from build123d import *

# Parameters (mm, degrees)
CYLINDER1785_R     = 5
CYLINDER1785_DEPTH = 3
CYLINDER1786_R     = 2.5
CYLINDER1786_DEPTH = 20
CYLINDER1781_R     = 1.5
CYLINDER1781_DEPTH = 20
CYLINDER1783_R     = 1.5
CYLINDER1783_DEPTH = 20
CYLINDER1784_R     = 1.5
CYLINDER1784_DEPTH = 20
CYLINDER1782_R     = 1.5
CYLINDER1782_DEPTH = 20
BOX744_W           = 6
BOX744_H           = 6
BOX744_DEPTH       = 2
BOX746_W           = 6
BOX746_H           = 6
BOX746_DEPTH       = 2
BOX745_W           = 6
BOX745_H           = 6
BOX745_DEPTH       = 2
BOX742_W           = 6
BOX742_H           = 6
BOX742_DEPTH       = 2
BOX743_W           = 20
BOX743_H           = 80
BOX743_DEPTH       = 20
BOX747_W           = 38
BOX747_H           = 32
BOX747_DEPTH       = 26
CHAMFER060_SIZE    = 2


with BuildPart() as obj1:
    # Cylinder1785 → Cylinder1785 (new body)
    with BuildSketch(Plane(origin=(-112, 16, 66), x_dir=(0, 0, -1), z_dir=(1, 0, 0))):
        Circle(CYLINDER1785_R)
    extrude(amount=CYLINDER1785_DEPTH)


with BuildPart() as obj2:
    # Cylinder1786 → Cylinder1786 (new body)
    with BuildSketch(Plane(origin=(-117, 16, 66), x_dir=(0, 0, -1), z_dir=(1, 0, 0))):
        Circle(CYLINDER1786_R)
    extrude(amount=CYLINDER1786_DEPTH)


with BuildPart() as obj3:
    # Cylinder1781 → Cylinder1781 (new body)
    with BuildSketch(Plane(origin=(-83, 25, 54), x_dir=(1, 0, 0), z_dir=(0, 0, 1))):
        Circle(CYLINDER1781_R)
    extrude(amount=CYLINDER1781_DEPTH)


with BuildPart() as obj4:
    # Cylinder1783 → Cylinder1783 (new body)
    with BuildSketch(Plane(origin=(-109, 7, 54), x_dir=(1, 0, 0), z_dir=(0, 0, 1))):
        Circle(CYLINDER1783_R)
    extrude(amount=CYLINDER1783_DEPTH)


with BuildPart() as obj5:
    # Cylinder1784 → Cylinder1784 (new body)
    with BuildSketch(Plane(origin=(-109, 25, 54), x_dir=(1, 0, 0), z_dir=(0, 0, 1))):
        Circle(CYLINDER1784_R)
    extrude(amount=CYLINDER1784_DEPTH)


with BuildPart() as compound913:
    # Cylinder1782 → Cylinder1782 (new body)
    with BuildSketch(Plane(origin=(-83, 7, 54), x_dir=(1, 0, 0), z_dir=(0, 0, 1))):
        Circle(CYLINDER1782_R)
    extrude(amount=CYLINDER1782_DEPTH)

    # Compound913: union obj3, obj4, obj5
    add(obj3.part)
    add(obj4.part)
    add(obj5.part)


with BuildPart() as krychle744:
    # Box744 → Box744 (new body)
    with BuildSketch(Plane(origin=(-112, 22, 60), x_dir=(1, 0, 0), z_dir=(0, 0, 1))):
        with Locations((3, 3)):
            Rectangle(BOX744_W, BOX744_H)
    extrude(amount=BOX744_DEPTH)


with BuildPart() as krychle746:
    # Box746 → Box746 (new body)
    with BuildSketch(Plane(origin=(-86, 4, 60), x_dir=(1, 0, 0), z_dir=(0, 0, 1))):
        with Locations((3, 3)):
            Rectangle(BOX746_W, BOX746_H)
    extrude(amount=BOX746_DEPTH)


with BuildPart() as krychle745:
    # Box745 → Box745 (new body)
    with BuildSketch(Plane(origin=(-86, 22, 60), x_dir=(1, 0, 0), z_dir=(0, 0, 1))):
        with Locations((3, 3)):
            Rectangle(BOX745_W, BOX745_H)
    extrude(amount=BOX745_DEPTH)


with BuildPart() as compound912:
    # Box742 → Box742 (new body)
    with BuildSketch(Plane(origin=(-112, 4, 60), x_dir=(1, 0, 0), z_dir=(0, 0, 1))):
        with Locations((3, 3)):
            Rectangle(BOX742_W, BOX742_H)
    extrude(amount=BOX742_DEPTH)

    # Compound912: union Krychle744, Krychle746, Krychle745
    add(krychle744.part)
    add(krychle746.part)
    add(krychle745.part)


with BuildPart() as krychle743:
    # Box743 → Box743 (new body)
    with BuildSketch(Plane(origin=(-106, 4, 56), x_dir=(1, 0, 0), z_dir=(0, 0, 1))):
        with Locations((10, 40)):
            Rectangle(BOX743_W, BOX743_H)
    extrude(amount=BOX743_DEPTH)


with BuildPart() as chamfer060:
    # Box747 → Box747 (new body)
    with BuildSketch(Plane(origin=(-112, 0, 56), x_dir=(1, 0, 0), z_dir=(0, 0, 1))):
        with Locations((19, 16)):
            Rectangle(BOX747_W, BOX747_H)
    extrude(amount=BOX747_DEPTH)

    # Cut546: cut Krychle743
    add(krychle743.part, mode=Mode.SUBTRACT)

    # Cut547: cut Compound912
    add(compound912.part, mode=Mode.SUBTRACT)

    # Cut541: cut Compound913
    add(compound913.part, mode=Mode.SUBTRACT)

    # Cut542: cut obj2
    add(obj2.part, mode=Mode.SUBTRACT)

    # Cut543: cut obj1
    add(obj1.part, mode=Mode.SUBTRACT)

    # Chamfer060
    chamfer060_edges = [chamfer060.edges().sort_by_distance(p)[0] for p in [
        (-112, 32, 69),
    ]]
    chamfer(chamfer060_edges, length=CHAMFER060_SIZE)


with BuildPart() as chamfer060_1:
    # Chamfer060 placement: moved
    add(chamfer060.part.moved(Location((0, 0, 2))))


solid = chamfer060_1.part
For this review, take the finished solid that the model builds, in its own axes (mm). A direction names the side the tool comes from. Round coordinates to 2 decimals unless told otherwise and drop trailing zeros. Write each loop counter-clockwise with the first axis right and the second up, starting at its lowest first coordinate (ties: lowest second). Pieces come first, ordered by that corner, then holes. Notation, with made-up numbers: (88.25, -38.5) -> (137.25, -38.5) arc R20 ccw to (137.25, -33.5) -> close; hole circle Ø10 at (89, 56). An arc over 180 degrees is marked (long way). Use CSV: the item, a comma, the result in double quotes.
(1) Consider section D-D, the plane y = 16. Give the boundary of the cut face in (x, z), plus the area to 3 significant figures.
Computed values:
outline,"(-112, 58) -> (-106, 58) -> (-106, 65.5) -> (-109, 65.5) -> (-109, 63) -> (-112, 63) -> close; (-112, 73) -> (-109, 73) -> (-109, 70.5) -> (-106, 70.5) -> (-106, 78) -> (-86, 78) -> (-86, 58) -> (-74, 58) -> (-74, 84) -> (-112, 84) -> close"
area,"543 mm²"
(2) Clearance check with flat-ended pins moving along their axes: P1, Ø2, axis at y = 15.5, z = 67.5, coming from the -X side; P2, Ø2.5, axis at x = -109, y = 25, coming from the -Z side; P3, Ø9, axis at y = 16, z = 68, coming from the -X side. State where each tip first meets the part, or that it passes through.
Computed values:
P1,"x = -86"
P2,"z = 76"
P3,"x = -109"
(3) For faces 1 (the face through (-84.4, 26.4, 64)), 2 (the face through (-86, 18, 68)), 3 (the face through (-110.5, 7.07, 59.97)), 4 (the face through (-93, 16, 84)), list the 3-axis set-ups (+Z, -Z, +X, -X, +Y, -Y) from which the entire face can be reached by the end or side of a thin tool; tool diameter is ignored.
Computed values:
face 1,"-X"
face 2,"-Z, +Y"
face 3,"-Z"
face 4,"+Z, +X, -X, +Y, -Y"
(4) To check wall thickness, follow L1, parallel to X at y = 25, z = 59.6; L2, parallel to Y at x = -109, z = 59.65; L3, parallel to X at y = 13.5, z = 75. State the ranges of each line that lie inside material, in increasing order. Write a range as [from, to].
Computed values:
L1,"[-112, -110.5], [-107.5, -106], [-86, -84.5], [-81.5, -74]"
L2,"[0, 5.5], [8.5, 23.5], [26.5, 32]"
L3,"[-112, -106], [-86, -74]"
(5) Consider section A-A, the plane z = 68. Give the boundary of the cut face in (x, y), plus the area to 3 significant figures.
Computed values:
outline,"(-112, 0) -> (-74, 0) -> (-74, 32) -> (-86, 32) -> (-86, 4) -> (-106, 4) -> (-106, 13.5) -> (-109, 13.5) -> (-109, 11) -> (-112, 11) -> close; (-112, 21) -> (-109, 21) -> (-109, 18.5) -> (-106, 18.5) -> (-106, 32) -> (-110, 32) -> (-112, 30) -> close; hole circle Ø3 at (-109, 7); hole circle Ø3 at (-109, 25); hole circle Ø3 at (-83, 7); hole circle Ø3 at (-83, 25)"
area,"581 mm²"
(6) Draft analysis for pull direction X (two halves, no side actions). For faces 5 (the face through (-112, 15, 74)), 6 (the face through (-82.194, 26.265, 59.972)), 7 (the face through (-109, 10, 63)), state which applies: +X half, -X half, draft (parallel to the pull), parting line (faces both ways), or undercut.
Computed values:
face 5,"-X half"
face 6,"undercut"
face 7,"draft"
(7) Consider section B-B, the plane y = 7. Give the number of separate pieces and of enclosed holes in the cut face, plus the area to 3 significant figures.
Computed values:
separate pieces,"4"
enclosed holes,"0"
area,"468 mm²"
(8) Consider section C-C, the plane x = -83. Give the boundary of the cut face in (y, z).
Computed values:
outline,"(0, 58) -> (5.5, 58) -> (5.5, 62) -> (4, 62) -> (4, 64) -> (5.5, 64) -> (5.5, 76) -> (8.5, 76) -> (8.5, 64) -> (10, 64) -> (10, 62) -> (8.5, 62) -> (8.5, 58) -> (23.5, 58) -> (23.5, 62) -> (22, 62) -> (22, 64) -> (23.5, 64) -> (23.5, 76) -> (26.5, 76) -> (26.5, 64) -> (28, 64) -> (28, 62) -> (26.5, 62) -> (26.5, 58) -> (32, 58) -> (32, 84) -> (0, 84) -> close"
